from build123d import *

# Parameters (mm, degrees)
RUN_START          = -20
SKETCH1_R          = 6
RUN_DEPTH          = 40
SKETCH2_R          = 6
BRANCH_DEPTH       = 25
SKETCH3_R          = 4
SUPPORT_POST_DEPTH = 20
SKETCH4_W          = 20
SKETCH4_H          = 20
SUPPORT_FOOT_DEPTH = 2


with BuildPart() as part:
    # Sketch1 → Run (new body)
    with BuildSketch(Plane(origin=(0, 0, 0), x_dir=(0, 0, -1), z_dir=(1, 0, 0)).offset(RUN_START)):
        with Locations((0, 25)):
            Circle(SKETCH1_R)
    extrude(amount=RUN_DEPTH)

    # Sketch2 → Branch (add)
    with BuildSketch(Plane.XY):
        with Locations(Location((0, 25, 0), (0, 0, 90))):
            Circle(SKETCH2_R)
    extrude(amount=BRANCH_DEPTH)

    # Sketch3 → Support_Post (add)
    with BuildSketch(Plane(origin=(0, 0, 0), x_dir=(1, 0, 0), z_dir=(0, 1, 0))):
        with Locations(Location((0, 0, 0), (0, 0, 123.987843581))):
            Circle(SKETCH3_R)
    extrude(amount=SUPPORT_POST_DEPTH)

    # Sketch4 → Support_Foot (add)
    with BuildSketch(Plane(origin=(0, 0, 0), x_dir=(1, 0, 0), z_dir=(0, 1, 0))):
        Rectangle(SKETCH4_W, SKETCH4_H)
    extrude(amount=SUPPORT_FOOT_DEPTH)


solid = part.part
Design review of the part built by this model. Coordinates are the model's own, in mm. A direction names the side the tool comes from. Give positions to 0.01 mm unless a question says otherwise; leave off trailing zeros. Loops run counter-clockwise (first coordinate to the right, second up) from the corner with the lowest first, then second, coordinate; pieces in that order, holes last. Notation, with made-up numbers: M -18,74 L -5,74 A16 ccw -5,96 Z; hole C 29,-15.75 d3. An arc over 180 degrees is marked long. One line per question, with ' | ' between items. Start each with the question number.
1. Insertion check: P1, Ø2, axis at x = -14.5, z = -2.5, coming from the -Y side; P2, Ø6, axis at x = -2, z = 20, coming from the -Y side; P3, Ø1, axis at x = -1, y = 3.5, coming from the +Z side. Each pin has a flat end and moves straight along its axis. Give the tip position at first contact, or say it passes through.
2. For faces 1 (the face through (4.3, 2, -0.1)), 2 (the face through (0, 1, 10)), 3 (the face through (5.323, 27.769, 15.103)), list the 3-axis set-ups (+Z, -Z, +X, -X, +Y, -Y) from which the entire face can be reached by the end or side of a thin tool; tool diameter is ignored.
3. To check wall thickness, follow L1, parallel to Y at x = -6, z = 0; L2, parallel to X at y = 25, z = 10. State the ranges of each line that lie inside material, in increasing order.
4. Add section C-C (z = -2.5). Write out the cut boundary in (x, y).
5. Add section D-D (x = 3.5). Write out the cut boundary in (y, z).
6. Add section A-A (x = 8.5). Write out the cut boundary in (y, z), plus the area to 3 significant figures.
7. Add section B-B (y = 25). Write out the cut boundary in (x, z), plus the area to 3 significant figures.
8. The part is to be moulded in two halves that separate along Y. For faces 4 (the face through (0, 25, 25)), 5 (the face through (-0.28, 26.802, -5.723)), 6 (the face through (0, 0, 0)), say which applies: released by +Y, released by -Y, zero draft, split by the parting line, or undercut.
Worked out:
1) P1: stops at y = 19.19 | P2: stops at y = 19 | P3: stops at z = 3.97
2) face 1: none | face 2: +Z, +X, -X, -Y | face 3: +Z
3) L1: y = 0 to 2, 19 to 31 | L2: x = -6 to 6
4) outline: M -20,19.55 L -3.12,19.55 L -3.12,2 L -10,2 L -10,0 L 10,0 L 10,2 L 3.12,2 L 3.12,19.55 L 20,19.55 L 20,30.45 L -20,30.45 Z
5) outline: M 0,-10 L 2,-10 L 2,-1.94 L 19.32,-1.94 A6 ccw long 29.87,3.5 L 29.87,25 L 20.13,25 L 20.13,3.5 A6 ccw 19.32,1.94 L 2,1.94 L 2,10 L 0,10 Z
6) outline: M 0,-10 L 2,-10 L 2,10 L 0,10 Z; C 25,0 d12 | area: 153 mm²
7) outline: M -20,-6 L 20,-6 L 20,6 L 6,6 L 6,25 L -6,25 L -6,6 L -20,6 Z | area: 708 mm²
8) face 4: zero draft | face 5: undercut | face 6: released by -Y
